Here's how the part is built. I have some questions about the finished solid (model axes, mm). Face numbers are marked on the shaded views. A direction names the side the tool comes from. Round coordinates to 2 decimals unless told otherwise and drop trailing zeros. Write each loop counter-clockwise with the first axis right and the second up, starting at its lowest first coordinate (ties: lowest second). Pieces come first, ordered by that corner, then holes. Notation, with made-up numbers: (29.25, -34.75) - (65.25, -34.75) arc R20 cw to (65.25, -27.75) - close; hole circle Ø9 at (19.5, 56.25). An arc over 180 degrees is marked (long way). Write item = value, one per line. Start each with the question number.
Item 1: If I drill on line 1 along Y through (x, z) = (-23, 12.25); line 2 along Z through (x, y) = (18, 26); line 3 along Z through (x, y) = (-36.5, 19), over which ranges is the centre line in solid material (lowest first)? Write a range as [from, to].
Item 2: For P1, Ø1.8, axis at x = 42.5, z = 0.5, coming from the -Y side; P2, Ø3, axis at x = -32, z = 3, coming from the +Y side; P3, Ø0.7, axis at x = 19, z = -1.5, coming from the +Y side, each with a flat end and sliding along its axis, tell me the tip position at first contact or that it passes through.
Item 3: If we section it at D-D (x = -13): Please give me the cut outline in (y, z).
Item 4: Which directions (+Z, -Z, +X, -X, +Y, -Y) give clear straight access to the entire face, cutting with the end or side of a thin tool? Please do the marked faces 5, 6, 7 and 8.
Item 5: Thinking about a two-plate mould opening in Y: for the marked faces 1, 2, 3 and 4, which applies, pulls with the +Y half, pulls with the -Y half, needs draft (parallel to the pull), parting line crosses it, or undercut?
Item 6: If we section it at B-B (z = 10): Please give me the cut outline in (x, y).
Item 7: If we section it at A-A (x = 17): Please give me the cut outline in (y, z) (3 decimals), and give its area (3 significant figures).
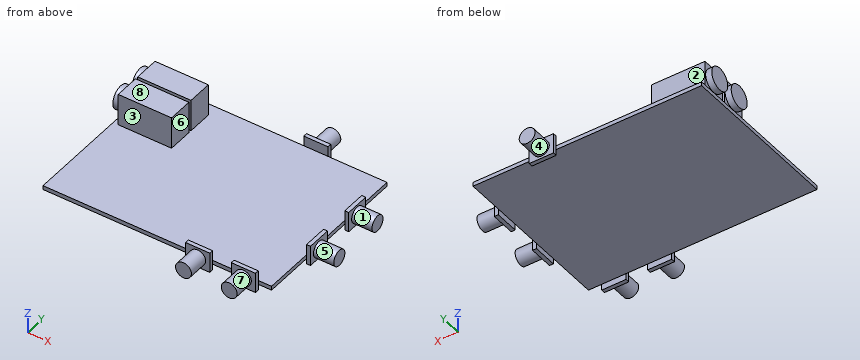
Autodesk Inventor part; units mm, degrees
ref_plane "YZ Plane" through (0, 0, 0) normal (1, 0, 0) x (0, 1, 0)
ref_plane "XZ Plane" through (0, 0, 0) normal (0, 1, 0) x (-1, 0, 0)
ref_plane "XY Plane" through (0, 0, 0) normal (0, 0, 1) x (1, 0, 0)
sketch "Sketch1" plane through (0, 0, 0) normal (0, 0, 1) x (1, 0, 0)
  line L0 (-45, 32.5) -> (45, 32.5)
  line L1 (45, 32.5) -> (45, -32.5)
  line L2 (45, -32.5) -> (-45, -32.5)
  line L3 (-45, -32.5) -> (-45, 32.5)
  line L4 (-45, 32.5) -> (45, -32.5) construction
  line L5 (45, 32.5) -> (-45, -32.5) construction
  point P0 (0, 0)
  dimension "d0" = 90
  dimension "d1" = 65
extrude "Extrusion1" add sketch "Sketch1" along normal blind 1.6
sketch "Sketch2" plane through (0, 0, 1.6) normal (0, 0, 1) x (1, 0, 0)
  point P0 (0, 0)
sketch "Sketch3" plane through (-45, 32.5, 0) normal (0, 1, 0) x (1, 0, 0)
  point P0 (45, 0)
sketch "Sketch4" plane through (-45, 32.5, 0) normal (0, 1, 0) x (1, 0, 0)
  line L0 (57.225, -5.6) -> (66.775, -5.6)
  line L1 (66.775, -5.6) -> (66.775, 2.4)
  line L2 (66.775, 2.4) -> (57.225, 2.4)
  line L3 (57.225, 2.4) -> (57.225, -5.6)
  line L4 (90, -1.6) -> (0, -1.6)
  line L5 (57.225, -5.6) -> (66.775, 2.4) construction
  line L6 (66.775, -5.6) -> (57.225, 2.4) construction
  point P0 (45, 0)
  point P1 (62, -1.6)
  dimension "d4" = 9.55
  dimension "d5" = 8
  dimension "d8" = 62
extrude "Extrusion2" add sketch "Sketch4" along normal blind 1.55
sketch "Sketch5" plane through (45, -32.5, 0) normal (1, 0, 0) x (0, 0, -1)
  line L0 (-5.6, 50.775) -> (2.4, 50.775)
  line L1 (2.4, 50.775) -> (2.4, 41.225)
  line L2 (2.4, 41.225) -> (-5.6, 41.225)
  line L3 (-5.6, 41.225) -> (-5.6, 50.775)
  line L4 (-1.6, 0) -> (-1.6, 65)
  line L5 (-5.6, 50.775) -> (2.4, 41.225) construction
  line L6 (2.4, 50.775) -> (-5.6, 41.225) construction
  line L7 (-5.8505, 29.275) -> (2.1495, 29.275)
  line L8 (2.1495, 29.275) -> (2.1495, 19.725)
  line L9 (2.1495, 19.725) -> (-5.8505, 19.725)
  line L10 (-5.8505, 19.725) -> (-5.8505, 29.275)
  line L11 (-5.8505, 29.275) -> (2.1495, 19.725) construction
  line L12 (2.1495, 29.275) -> (-5.8505, 19.725) construction
  point P0 (0, 32.5)
  point P1 (-1.6, 46)
  point P2 (-1.8505, 24.5)
  dimension "d9" = 9.55
  dimension "d10" = 8
  dimension "d11" = 19
  dimension "d12" = 24.5
extrude "Extrusion3" add sketch "Sketch5" along normal blind 1.55
sketch "Sketch6" plane through (-45, -32.5, 0) normal (0, -1, 0) x (1, 0, 0)
  line L0 (66.775, 5.6091) -> (57.225, 5.6091)
  line L1 (57.225, 5.6091) -> (57.225, -2.3909)
  line L2 (57.225, -2.3909) -> (66.775, -2.3909)
  line L3 (66.775, -2.3909) -> (66.775, 5.6091)
  line L4 (66.775, 5.6091) -> (57.225, -2.3909) construction
  line L5 (57.225, 5.6091) -> (66.775, -2.3909) construction
  line L6 (84.775, 5.6) -> (75.225, 5.6)
  line L7 (75.225, 5.6) -> (75.225, -2.4)
  line L8 (75.225, -2.4) -> (84.775, -2.4)
  line L9 (84.775, -2.4) -> (84.775, 5.6)
  line L10 (0, 1.6) -> (90, 1.6)
  line L11 (84.775, 5.6) -> (75.225, -2.4) construction
  line L12 (75.225, 5.6) -> (84.775, -2.4) construction
  point P0 (45, 0)
  point P1 (62, 1.6091)
  point P2 (80, 1.6)
  dimension "d15" = 10
  dimension "d16" = 28
  dimension "d17" = 8
  dimension "d18" = 9.55
extrude "Extrusion4" add sketch "Sketch6" along normal blind 1.55
sketch "Sketch7" plane through (0, 0, 1.6) normal (0, 0, 1) x (1, 0, 0)
  line L0 (-43, 27.7) -> (-22, 27.7)
  line L1 (-22, 27.7) -> (-22, 17.95)
  line L2 (-22, 17.95) -> (-43, 17.95)
  line L3 (-43, 17.95) -> (-43, 27.7)
  line L4 (-43, 27.7) -> (-22, 17.95) construction
  line L5 (-22, 27.7) -> (-43, 17.95) construction
  line L6 (-43, 16.75) -> (-22, 16.75)
  line L7 (-22, 16.75) -> (-22, 7)
  line L8 (-22, 7) -> (-43, 7)
  line L9 (-43, 7) -> (-43, 16.75)
  line L10 (-43, 16.75) -> (-22, 7) construction
  line L11 (-22, 16.75) -> (-43, 7) construction
  line L12 (12.225, 32.5) -> (-45, 32.5)
  line L13 (-45, 32.5) -> (-45, -32.5)
  point P0 (0, 0)
  point P1 (-32.5, 22.825)
  point P2 (-32.5, 11.875)
  dimension "d21" = 21
  dimension "d22" = 9.75
  dimension "d23" = 25.5
  dimension "d24" = 4.8
  dimension "d25" = 2
extrude "Extrusion5" add sketch "Sketch7" along normal blind 12.6
sketch "Sketch8" plane through (-43, 17.95, 1.6) normal (-1, 0, 0) x (0, 0, 1)
  circle A0 centre (7.3783, 4.875) radius 4.5
  circle A1 centre (7.3783, -6.0762) radius 4.5
  point P0 (-1.6, -17.95)
  dimension "d28" = 9
extrude "Extrusion6" add sketch "Sketch8" along normal blind 2.4
sketch "Sketch9" plane through (-45, -34.05, 0) normal (0, -1, 0) x (1, 0, 0)
  line L0 (66.775, 5.6091) -> (57.225, 5.6091) construction
  line L1 (62, 5.6091) -> (62, -2.3909) construction
  line L2 (57.225, -2.3909) -> (66.775, -2.3909) construction
  line L3 (57.225, 1.6) -> (66.775, 1.6) construction
  line L4 (57.225, 1.6) -> (66.775, 1.6) construction
  line L5 (84.775, 5.6) -> (75.225, 5.6) construction
  line L6 (80, 5.6) -> (80, -3.4898) construction
  line L7 (75.225, 0) -> (75.225, 1.6) construction
  line L8 (75.225, 1.6) -> (84.775, 1.6) construction
  line L9 (75.225, 1.6) -> (84.775, 1.6) construction
  circle A0 centre (62, 1.6) radius 3.125
  circle A1 centre (80, 1.6) radius 3.125
  point P0 (45, 0)
  dimension "d31" = 6.25
extrude "Extrusion7" add sketch "Sketch9" along normal blind 8
sketch "Sketch10" plane through (46.55, -32.5, 0) normal (1, 0, 0) x (0, 0, -1)
  line L0 (-5.6, 50.775) -> (-5.6, 41.225) construction
  line L1 (-5.6, 46) -> (2.4, 46) construction
  line L2 (2.4, 41.225) -> (2.4, 50.775) construction
  line L3 (-5.8505, 29.275) -> (-5.8505, 19.725) construction
  line L4 (-5.8505, 24.5) -> (2.1495, 24.5) construction
  line L5 (2.1495, 29.275) -> (2.1495, 19.725) construction
  line L6 (-1.6, 50.775) -> (0, 50.775) construction
  line L7 (-1.6, 39.5) -> (-1.6, 49.25) construction
  line L8 (-1.6, 50.775) -> (-1.6, 39.5) construction
  line L9 (-1.6, 65) -> (-1.6, 0) construction
  line L10 (-1.6, 29.275) -> (-1.6, 19.725) construction
  circle A0 centre (-1.6, 46) radius 3.125
  circle A1 centre (-1.6, 24.5) radius 3.125
  point P0 (0, 32.5)
  dimension "d34" = 6.25
extrude "Extrusion8" add sketch "Sketch10" along normal blind 8
sketch "Sketch11" plane through (-45, 34.05, 0) normal (0, 1, 0) x (1, 0, 0)
  line L0 (66.775, -5.6091) -> (57.225, -5.6091) construction
  line L1 (62, -5.6091) -> (62, 2.3909) construction
  line L2 (57.225, 2.3909) -> (66.775, 2.3909) construction
  line L3 (57.225, -1.6) -> (66.775, -1.6) construction
  line L4 (57.225, -1.6) -> (66.775, -1.6) construction
  circle A0 centre (62, -1.6) radius 3.125
  point P0 (45, 0)
  dimension "d37" = 6.25
extrude "Extrusion9" add sketch "Sketch11" along normal blind 8
properties part number "ADF41020-EVB"
Reply:
q1.line_1 = [7, 16.75], [17.95, 27.7]
q1.line_2 = [0, 1.6]
q1.line_3 = [0, 14.2]
q2.P1 = -32.5
q2.P2 = 32.5
q2.P3 = 34.05
q3.outline = (-32.5, 0) - (32.5, 0) - (32.5, 1.6) - (-32.5, 1.6) - close
q4.face_5 = +X
q4.face_6 = +Z, +Y, -Y
q4.face_7 = -Y
q4.face_8 = +Z, +X, -X, +Y, -Y
q5.face_1 = undercut
q5.face_2 = pulls with the +Y half
q5.face_3 = pulls with the -Y half
q5.face_4 = needs draft
q6.outline = (-45.4, 7.49) - (-43, 7.49) - (-43, 7) - (-22, 7) - (-22, 16.75) - (-43, 16.75) - (-43, 16.26) - (-45.4, 16.26) - close; (-45.4, 18.44) - (-43, 18.44) - (-43, 17.95) - (-22, 17.95) - (-22, 27.7) - (-43, 27.7) - (-43, 27.21) - (-45.4, 27.21) - close
q7.outline = (-42.05, -1.525) - (-34.05, -1.525) - (-34.05, -2.391) - (-32.5, -2.391) - (-32.5, 0) - (32.5, 0) - (32.5, -2.4) - (34.05, -2.4) - (34.05, -1.525) - (42.05, -1.525) - (42.05, 4.725) - (34.05, 4.725) - (34.05, 5.6) - (32.5, 5.6) - (32.5, 1.6) - (-32.5, 1.6) - (-32.5, 5.609) - (-34.05, 5.609) - (-34.05, 4.725) - (-42.05, 4.725) - close
q7.area = 229 mm2
